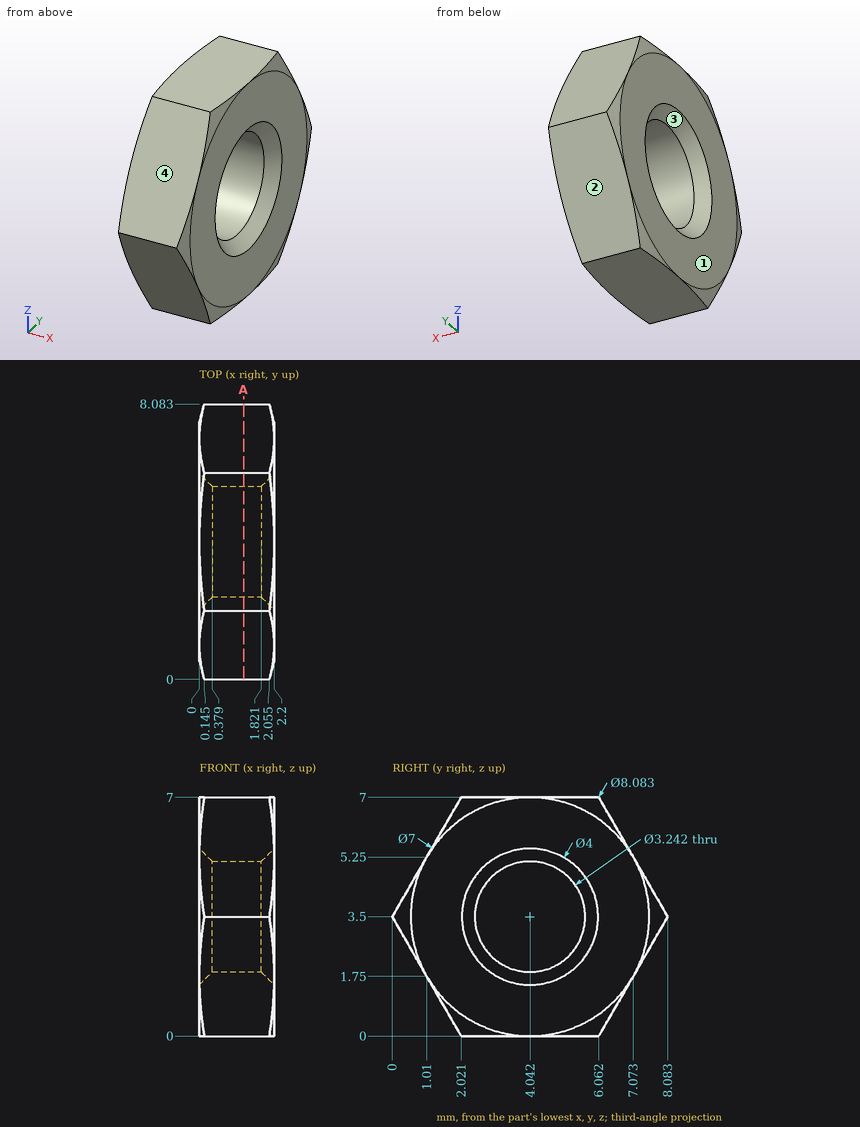
Study the drawing (mm; zero at the part's minimum x, y, z) and answer. Give positions to 0.01 mm unless a question says otherwise; leave off trailing zeros. Order: outer loops, then holes, each group sorted by start corner. A loop starts at its lowest first (then second) coordinate and runs counter-clockwise, first axis right, second up. Notation, with made-up numbers: (73.25, 43.25) -> (118.25, 43.25) arc R15 ccw to (118.25, 71.25) -> close; hole circle Ø2 at (-29.5, 76.5). An arc over 180 degrees is marked (long way). Put each result on its own line as item: value.
Item 1: Given P1, Ø1.5, axis at y = 5, z = 3, coming from the +X side, flat-ended and moving along its own axis, determine where the tip first touches the part or whether it passes through.
Established:
P1: stops at x = 2.03
Item 2: For a pull along Z with two mould halves and no side action, classify the marked faces 1, 2, 3 and 4 as released by +Z, released by -Z, zero draft, split by the parting line, or undercut.
Established:
face 1: zero draft
face 2: released by -Z
face 3: undercut
face 4: released by +Z
Item 3: A cutting plane is placed at A-A on x = 1.3. Give the vertices of the cut face in (y, z).
Established:
outline: (0, 3.5) -> (2.02, 0) -> (6.06, 0) -> (8.08, 3.5) -> (6.06, 7) -> (2.02, 7) -> close; hole circle Ø3.24 at (4.04, 3.5)
Item 4: Straight lines are drawn through the part: line 1 (Z direction, x = 0.7, y = 4.25); line 2 (Z direction, x = 0.4, y = 4.75); line 3 (Y direction, x = 1.25, z = 4.5) (1 decimal). For each, find the intervals that lie inside material, in ascending order.
Established:
line 1: z = 0 to 1.89, 5.11 to 7
line 2: z = 0 to 2.04, 4.96 to 7
line 3: y = 0.6 to 2.8, 5.3 to 7.5
